```python
from build123d import *

# Parameters (mm, degrees)
F1_DEPTH = 19.05
F3_DEPTH = 25.4


with BuildPart() as f1:
    # F0 (on Top) → F1 (new body)
    with BuildSketch(Plane.XY):
        Polygon((38.729571, 51.290266), (-27.945429, 51.290266), (-27.945429, -37.609734), (-9.614558, -69.359734), (-2.545429, -69.359734), (-2.545429, -12.209734), (13.329571, -12.209734), (13.329571, -69.359734), (20.3987, -69.359734), (38.729571, -37.609734), align=None)
    extrude(amount=F1_DEPTH)

    # F2 (on face) → F3 (join)
    with BuildSketch(Plane(origin=(0, 51.290266, 0), x_dir=(-1, 0, 0), z_dir=(0, 1, 0))):
        Polygon((-38.729571, 44.45), (-38.729571, 19.05), (27.945429, 19.05), (27.945429, 44.45), (1.563081, 44.45), (8.895429, 31.75), (-19.679571, 31.75), (-12.347222, 44.45), align=None)
    extrude(amount=-F3_DEPTH)


solid = f1.part
```
Input: part model. Units: mm. Frame: model coordinates. A direction names the side the tool comes from. Give positions to 0.01 mm unless a question says otherwise; leave off trailing zeros. Order: outer loops, then holes, each group sorted by start corner. A loop starts at its lowest first (then second) coordinate and runs counter-clockwise, first axis right, second up.
1. Material intervals for L1, parallel to Z at x = 5.5, y = 29; L2, parallel to X at y = -57, z = 18; L3, parallel to Y at x = 30, z = 37.5, sorted ascending.
Derived:
L1: z = 0 to 31.75
L2: x = -16.75 to -2.55, 13.33 to 27.53
L3: y = 25.89 to 51.29
2. Pin query (flat end, axial travel): pin 1 (15 mm diameter, centred on y = -46, z = 8, fed in from +X); pin 2 (8 mm diameter, centred on x = 5.5, y = 1, fed in from +Z); pin 3 (5.5 mm diameter, centred on y = -46.5, z = 6, fed in from -X). Return the tip coordinate at first contact, or that it passes through.
Derived:
pin 1: stops at x = 38.22
pin 2: stops at z = 19.05
pin 3: stops at x = -24.4
3. Section C-C on x = 14.5. Return the cut outline in (y, z).
Derived:
outline: (-69.36, 0) - (51.29, 0) - (51.29, 31.75) - (25.89, 31.75) - (25.89, 19.05) - (-69.36, 19.05) - close; (25.89, 40.72) - (51.29, 40.72) - (51.29, 44.45) - (25.89, 44.45) - close
4. Section B-B on z = 5.5. Return the cut outline in (x, y), and give its area (3 significant figures).
Derived:
outline: (-27.95, -37.61) - (-9.61, -69.36) - (-2.55, -69.36) - (-2.55, -12.21) - (13.33, -12.21) - (13.33, -69.36) - (20.4, -69.36) - (38.73, -37.61) - (38.73, 51.29) - (-27.95, 51.29) - close
area: 6,560 mm2
5. Section A-A on y = -29.5. Return the cut outline in (x, z).
Derived:
outline: (-27.95, 0) - (-2.55, 0) - (-2.55, 19.05) - (-27.95, 19.05) - close; (13.33, 0) - (38.73, 0) - (38.73, 19.05) - (13.33, 19.05) - close
6. Reachability of faces 1 (the flat face through (5, -10, 19.05)), 2 (the flat face through (5, 39, 31.75)), 3 (the flat face through (5, -12.21, 9)) from +Z, -Z, +X, -X, +Y, -Y: full face, straight path, thin tool, end or side. Return the list, or none.
Derived:
face 1: +Z, +X, -X, -Y
face 2: +Y, -Y
face 3: +Z, -Z, -Y
7. Section D-D on x = 0. Return the cut outline in (y, z).
Derived:
outline: (-12.21, 0) - (51.29, 0) - (51.29, 31.75) - (25.89, 31.75) - (25.89, 19.05) - (-12.21, 19.05) - close
